Can you work these out from the drawing? Everything is in mm from the part's minimum corner. A direction names the side the tool comes from. Give positions to 0.01 mm unless a question says otherwise; leave off trailing zeros. Loops run counter-clockwise (first coordinate to the right, second up) from the corner with the lowest first, then second, coordinate; pieces in that order, holes last. Notation, with made-up numbers: (-18, 0) -> (-4, 0) arc R11 cw to (-4, 14) -> close; hole circle Ø5 at (-12, 26.5). An arc over 180 degrees is marked (long way). Write item = value, one per line. Start each with the question number.
1) I want a section at C-C (x = 381). List the corners of the cut face in (y, z) for me.
2) I want a section at B-B (y = 480.5). List the corners of the cut face in (x, z) for me, and give its area (3 significant figures).
3) I want a section at D-D (x = 604). List the corners of the cut face in (y, z) for me.
4) On a 3-axis mill with a long thin cutter (end or side, diameter ignored), from which of +Z, -Z, +X, -X, +Y, -Y can I reach the whole of each face in a straight line? I mean the marked faces 1, 2 and 3. Say none if no direction works.
5) I want a section at A-A (z = 428). List the corners of the cut face in (x, y) for me, and give its area (3 significant figures).
6) If we mould it in two halves opening along Z, with no side actions, what happens to the marked faces 4, 5, 6 and 7? For each: +Z half, -Z half, draft (parallel to the pull), parting line (faces both ways), or undercut.
7) I need wall thicknesses on probe 1 along Y at (x, z) = (306, 320.5); probe 2 along Z at (x, y) = (1131, 208.5); probe 3 along X at (y, z) = (109.5, 460.5). Which ranges of each line are inside material? Lowest first, please. Write a range as from..to.
8) I'm going to push flat-ended pins straight in: pin 1 Ø12 at (x, y) = (563.5, 143) entering from -Z; pin 2 Ø3 at (x, z) = (392.5, 318) entering from -Y. Where does each tip first touch, or does it pass through?
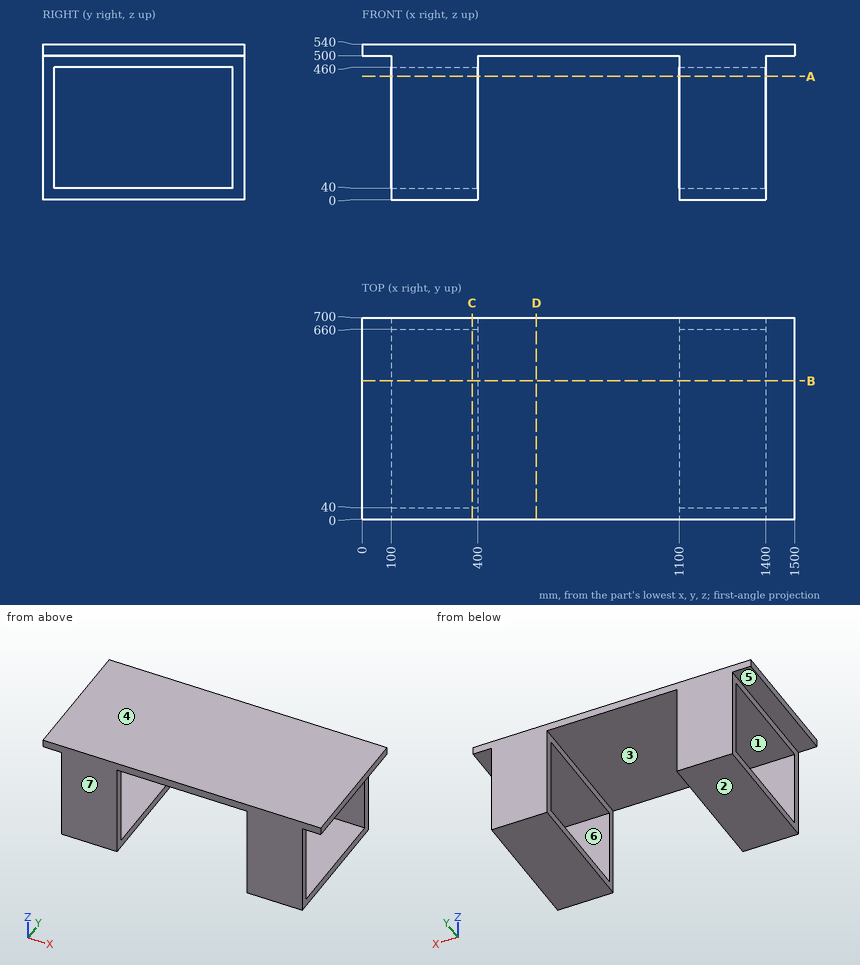
Answer list:
q1.outline = (0, 0) -> (700, 0) -> (700, 540) -> (0, 540) -> close; hole (40, 40) -> (660, 40) -> (660, 460) -> (40, 460) -> close
q2.outline = (0, 500) -> (100, 500) -> (100, 460) -> (400, 460) -> (400, 500) -> (1100, 500) -> (1100, 460) -> (1400, 460) -> (1400, 500) -> (1500, 500) -> (1500, 540) -> (0, 540) -> close; (100, 0) -> (400, 0) -> (400, 40) -> (100, 40) -> close; (1100, 0) -> (1400, 0) -> (1400, 40) -> (1100, 40) -> close
q2.area = 108,000 mm^2
q3.outline = (0, 500) -> (700, 500) -> (700, 540) -> (0, 540) -> close
q4.face_1 = +X, -X
q4.face_2 = -Z, +X, -X, +Y, -Y
q4.face_3 = -Z, +Y, -Y
q5.outline = (100, 0) -> (400, 0) -> (400, 40) -> (100, 40) -> close; (100, 660) -> (400, 660) -> (400, 700) -> (100, 700) -> close; (1100, 0) -> (1400, 0) -> (1400, 40) -> (1100, 40) -> close; (1100, 660) -> (1400, 660) -> (1400, 700) -> (1100, 700) -> close
q5.area = 48,000 mm^2
q6.face_4 = +Z half
q6.face_5 = -Z half
q6.face_6 = undercut
q6.face_7 = draft
q7.probe_1 = 0..40, 660..700
q7.probe_2 = 0..40, 460..540
q7.probe_3 = 100..400, 1100..1400
q8.pin_1 = 500
q8.pin_2 = 0
